Here's how the part is built. I have some questions about the finished solid (model axes, mm). Face numbers are marked on the shaded views. Round coordinates to 2 decimals unless told otherwise and drop trailing zeros. Loops run counter-clockwise (first coordinate to the right, second up) from the corner with the lowest first, then second, coordinate; pieces in that order, holes last. Notation, with made-up numbers: (75, 55.25) -> (104, 55.25) arc R23 ccw to (104, 79.25) -> close; hole circle Ø4 at (84.5, 69.25). An arc over 180 degrees is marked (long way). Use one line per item in the form item = value. Start each with the question number.
Item 1: Thinking about a two-plate mould opening in Z: for the marked faces 1 and 2, which applies, released by +Z, released by -Z, zero draft, split by the parting line, or undercut?
Item 2: If we section it at D-D (x = -5.25): Write out the boundary of the cut face in (y, z).
Item 3: I'm going to push flat-ended pins straight in: pin 1 Ø1 at (x, y) = (-1.5, 14) entering from +Z; pin 2 Ø3 at (y, z) = (-18.5, 32.04) entering from +X; pin 3 Ø10 at (y, z) = (-10, -17.32) entering from -X; pin 4 Ø5 at (x, y) = (-3.5, 13) entering from +Z. Where does each tip first touch, or does it pass through?
Item 4: If we section it at C-C (y = -8.5): Write out the boundary of the cut face in (x, z), then the cut area to 3 significant figures.
Item 5: If we section it at A-A (z = 0): Write out the boundary of the cut face in (x, y).
Item 6: If I drill on L1, parallel to Y at x = -0.7, z = 0; L2, parallel to Z at x = -1.75, y = -11.5; L3, parallel to Y at x = -6.25, z = 13, over which ranges is the centre line in solid material (lowest first)? Write a range as [from, to].
Item 7: If we section it at B-B (y = -18.5): Write out the boundary of the cut face in (x, z), then the cut area to 3 significant figures.
```python
from build123d import *

# Parameters (mm, degrees)
AXIAL_BLANK_PROFILE_W                          = 3
AXIAL_BLANK_PROFILE_H                          = 41
RELOCATED_START                                = -11
RELOCATED_INTEGRAL_PORT_BOSSES_BETWE_2_R       = 7
RELOCATED_INTEGRAL_PORT_BOSSES_BETWEEN_M_DEPTH = 8
SEVEN_START                                    = -3
SEVEN_DRY_MAGNET_PASSAGES_THROUGH_CO_2_R       = 6.3
SEVEN_DRY_MAGNET_PASSAGES_THROUGH_CO_2_R_2     = 4.3
SEVEN_DRY_MAGNET_PASSAGES_THROUGH_COVER_DEPTH  = 3
SIX_START                                      = -3
SIX_COVER_CLEARANCE_HOLES_PCD74_SKETCH_R       = 1.7
SIX_COVER_CLEARANCE_HOLES_PCD74_DEPTH          = 3
G1_8_START                                     = -11
G1_8_TAPPING_PILOT_ENVELOPES_DEPTH7_SKET_R     = 4.4
G1_8_TAPPING_PILOT_ENVELOPES_DEPTH7_DEPTH      = 7
WATER_START                                    = -11
WATER_PORTS_DIAMETER4_INTO_COOLANT_P_2_R       = 2
WATER_PORTS_DIAMETER4_INTO_COOLANT_PLENU_DEPTH = 11


with BuildPart() as part:
    # Axial blank profile → Native revolved blank (revolve)
    with BuildSketch(Plane.XY, mode=Mode.PRIVATE) as native_revolved_blank_sk:
        with Locations((-1.5, 20.5)):
            Rectangle(AXIAL_BLANK_PROFILE_W, AXIAL_BLANK_PROFILE_H)
    revolve(native_revolved_blank_sk.sketch.rotate(Axis((-60, 0, 0), (1, 0, 0)), 90), axis=Axis((-60, 0, 0), (1, 0, 0)))

    # Relocated integral port bosses betwe 2 → Relocated integral port bosses between m (add)
    with BuildSketch(Plane(origin=(0, 0, 0), x_dir=(0, 0, -1), z_dir=(1, 0, 0)).offset(RELOCATED_START)):
        with Locations((-13, 22.516660498)):
            Circle(RELOCATED_INTEGRAL_PORT_BOSSES_BETWE_2_R)
        with Locations((13, 22.516660498)):
            Circle(RELOCATED_INTEGRAL_PORT_BOSSES_BETWE_2_R)
    extrude(amount=RELOCATED_INTEGRAL_PORT_BOSSES_BETWEEN_M_DEPTH)

    # Seven dry magnet passages through co 2 → Seven dry magnet passages through cover (cut)
    with BuildSketch(Plane(origin=(0, 0, 0), x_dir=(0, 0, -1), z_dir=(1, 0, 0)).offset(SEVEN_START)):
        Circle(SEVEN_DRY_MAGNET_PASSAGES_THROUGH_CO_2_R)
        with Locations((0, 20)):
            Circle(SEVEN_DRY_MAGNET_PASSAGES_THROUGH_CO_2_R_2)
        with Locations((-17.320508076, 10)):
            Circle(SEVEN_DRY_MAGNET_PASSAGES_THROUGH_CO_2_R_2)
        with Locations((-17.320508076, -10)):
            Circle(SEVEN_DRY_MAGNET_PASSAGES_THROUGH_CO_2_R_2)
        with Locations((0, -20)):
            Circle(SEVEN_DRY_MAGNET_PASSAGES_THROUGH_CO_2_R_2)
        with Locations((17.320508076, -10)):
            Circle(SEVEN_DRY_MAGNET_PASSAGES_THROUGH_CO_2_R_2)
        with Locations((17.320508076, 10)):
            Circle(SEVEN_DRY_MAGNET_PASSAGES_THROUGH_CO_2_R_2)
    extrude(amount=SEVEN_DRY_MAGNET_PASSAGES_THROUGH_COVER_DEPTH, mode=Mode.SUBTRACT)

    # Six cover clearance holes PCD74 sketch → Six cover clearance holes PCD74 (cut)
    with BuildSketch(Plane(origin=(0, 0, 0), x_dir=(0, 0, -1), z_dir=(1, 0, 0)).offset(SIX_START)):
        with Locations((0, 37)):
            Circle(SIX_COVER_CLEARANCE_HOLES_PCD74_SKETCH_R)
        with Locations((-32.04293994, 18.5)):
            Circle(SIX_COVER_CLEARANCE_HOLES_PCD74_SKETCH_R)
        with Locations((-32.04293994, -18.5)):
            Circle(SIX_COVER_CLEARANCE_HOLES_PCD74_SKETCH_R)
        with Locations((0, -37)):
            Circle(SIX_COVER_CLEARANCE_HOLES_PCD74_SKETCH_R)
        with Locations((32.04293994, -18.5)):
            Circle(SIX_COVER_CLEARANCE_HOLES_PCD74_SKETCH_R)
        with Locations((32.04293994, 18.5)):
            Circle(SIX_COVER_CLEARANCE_HOLES_PCD74_SKETCH_R)
    extrude(amount=SIX_COVER_CLEARANCE_HOLES_PCD74_DEPTH, mode=Mode.SUBTRACT)

    # G1-8 tapping pilot envelopes depth7 sketch → G1-8 tapping pilot envelopes depth7 (cut)
    with BuildSketch(Plane(origin=(0, 0, 0), x_dir=(0, 0, -1), z_dir=(1, 0, 0)).offset(G1_8_START)):
        with Locations((-13, 22.516660498)):
            Circle(G1_8_TAPPING_PILOT_ENVELOPES_DEPTH7_SKET_R)
        with Locations((13, 22.516660498)):
            Circle(G1_8_TAPPING_PILOT_ENVELOPES_DEPTH7_SKET_R)
    extrude(amount=G1_8_TAPPING_PILOT_ENVELOPES_DEPTH7_DEPTH, mode=Mode.SUBTRACT)

    # Water ports diameter4 into coolant p 2 → Water ports diameter4 into coolant plenu (cut)
    with BuildSketch(Plane(origin=(0, 0, 0), x_dir=(0, 0, -1), z_dir=(1, 0, 0)).offset(WATER_START)):
        with Locations((-13, 22.516660498)):
            Circle(WATER_PORTS_DIAMETER4_INTO_COOLANT_P_2_R)
        with Locations((13, 22.516660498)):
            Circle(WATER_PORTS_DIAMETER4_INTO_COOLANT_P_2_R)
    extrude(amount=WATER_PORTS_DIAMETER4_INTO_COOLANT_PLENU_DEPTH, mode=Mode.SUBTRACT)


solid = part.part
```
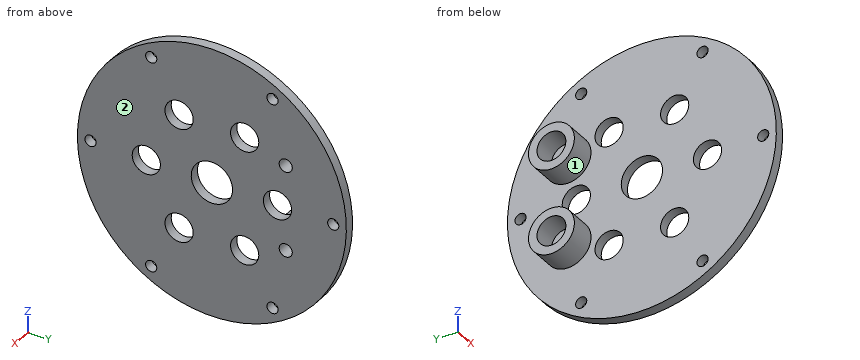
Values found:
q1.face_1 = undercut
q1.face_2 = zero draft
q2.outline = circle Ø14 at (22.52, -13); circle Ø14 at (22.52, 13); hole circle Ø8.8 at (22.52, -13); hole circle Ø8.8 at (22.52, 13)
q3.pin_1 = 38.71
q3.pin_2 = through
q3.pin_3 = -3
q3.pin_4 = 39.62
q4.outline = (-3, -40.11) -> (0, -40.11) -> (0, -21.35) -> (-3, -21.35) -> close; (-3, -13.29) -> (0, -13.29) -> (0, 13.29) -> (-3, 13.29) -> close; (-3, 21.35) -> (0, 21.35) -> (0, 40.11) -> (-3, 40.11) -> close
q4.area = 192 mm2
q5.outline = (-3, -41) -> (0, -41) -> (0, -38.7) -> (-3, -38.7) -> close; (-3, -35.3) -> (0, -35.3) -> (0, -24.3) -> (-3, -24.3) -> close; (-3, -15.7) -> (0, -15.7) -> (0, -6.3) -> (-3, -6.3) -> close; (-3, 6.3) -> (0, 6.3) -> (0, 15.7) -> (-3, 15.7) -> close; (-3, 24.3) -> (0, 24.3) -> (0, 35.3) -> (-3, 35.3) -> close; (-3, 38.7) -> (0, 38.7) -> (0, 41) -> (-3, 41) -> close
q6.L1 = [-41, -38.7], [-35.3, -24.3], [-15.7, -6.3], [6.3, 15.7], [24.3, 35.3], [38.7, 41]
q6.L2 = [-39.35, -21.35], [-13.29, 13.29], [21.35, 39.35]
q6.L3 = [15.52, 18.12], [26.92, 29.52]
q7.outline = (-3, -36.59) -> (0, -36.59) -> (0, -33.74) -> (-3, -33.74) -> close; (-3, -30.34) -> (0, -30.34) -> (0, -4.03) -> (-3, -4.03) -> close; (-3, 4.03) -> (0, 4.03) -> (0, 30.34) -> (-3, 30.34) -> close; (-3, 33.74) -> (0, 33.74) -> (0, 36.59) -> (-3, 36.59) -> close
q7.area = 175 mm2
